Verification items for the finished model (mm, model axes). A direction names the side the tool comes from. Coordinates: 2 decimals unless noted, no trailing zeros. Write each loop counter-clockwise with the first axis right and the second up, starting at its lowest first coordinate (ties: lowest second). Pieces come first, ordered by that corner, then holes.
Autodesk Inventor part; units mm, degrees
ref_plane "Work Plane4" through (0, 32, 0) normal (0, 1, 0) x (-1, 0, 0)
ref_plane "YZ Plane" through (0, 0, 0) normal (1, 0, 0) x (0, 1, 0)
ref_plane "XY Plane" through (0, 0, 0) normal (0, 0, 1) x (1, 0, 0)
ref_plane "Work Plane4" through (0, 32, 0) normal (0, 1, 0) x (-1, 0, 0)
sketch "Sketch1" plane through (0, 0, 0) normal (0, 1, 0) x (-1, 0, 0)
  line L0 (33.75, 44.75) -> (-33.75, 44.75)
  line L1 (-33.75, 44.75) -> (-33.75, -44.75)
  line L2 (-33.75, -44.75) -> (33.75, -44.75)
  line L3 (33.75, -44.75) -> (33.75, 44.75)
  line L4 (21.75, -36.75) -> (-21.75, -36.75)
  line L5 (21.75, 36.75) -> (-21.75, 36.75)
  line L6 (21.75, 36.75) -> (21.75, -36.75)
  line L7 (-21.75, 36.75) -> (-21.75, -36.75)
  line L8 (33.75, -41.75) -> (-33.75, -41.75)
  line L9 (33.75, 41.75) -> (-33.75, 41.75)
  line L10 (-6.7955, 36.75) -> (21.75, 0)
  line L11 (21.75, 0) -> (0, -36.75)
  point P0 (0, 0)
  point P1 (-33.75, 0)
  dimension "d0" = 83.5
  dimension "d1" = 3
  dimension "d2" = 3
  dimension "d4" = 5
  dimension "d5" = 5
  dimension "d6" = 12
  dimension "d7" = 12
  dimension "d8" = 67.5
  dimension "d9" = 33.75
  dimension "d10" = 41.75
sketch "Sketch2" plane through (0, 32, 0) normal (0, 1, 0) x (1, 0, 0)
  line L0 (-65.75, 34.75) -> (24.75, 34.75)
  line L1 (-65.75, -34.75) -> (24.75, -34.75)
  line L2 (24.75, -34.75) -> (24.75, 34.75)
  line L3 (-65.75, -34.75) -> (-65.75, 34.75)
  line L4 (-74.75, -44.75) -> (-74.75, 44.75)
  line L5 (33.75, -44.75) -> (33.75, 44.75)
  line L6 (33.75, 44.75) -> (-33.75, 44.75)
  line L7 (-74.75, -44.75) -> (33.75, -44.75)
  line L8 (-74.75, 44.75) -> (33.75, 44.75)
  dimension "d94" = 69.5
  dimension "d96" = 90.5
  dimension "d97" = 9
  dimension "d98" = 9
  dimension "d99" = 10
  dimension "d100" = 10
extrude "Extrusion3" add sketch "Sketch2" along normal blind 3
sketch "Sketch3" plane through (0, 32, 0) normal (0, 1, 0) x (1, 0, 0)
  circle A0 centre (29.25, 0) radius 4.5
  circle A1 centre (-70.45, 0) radius 4.5
  circle A2 centre (-70.45, 0) radius 2.35
  circle A3 centre (29.25, 0) radius 2.35
  line L0 (33.75, -44.75) -> (33.75, 44.75)
  point P0 (0, 0)
  dimension "d24" = 9
  dimension "d27" = 4.7
  dimension "d43" = 99.7
  dimension "d44" = 4.5
extrude "Extrusion5" cut sketch "Sketch3" along normal blind 3 contours A2 | A3
sketch "Sketch9" plane through (0, 35, 0) normal (0, 1, 0) x (1, 0, 0)
  circle A0 centre (-39, -50.75) radius 3
  circle A1 centre (-39, -50.75) radius 6
  line L0 (-74.75, -44.75) -> (33.75, -44.75)
  circle A2 centre (-2, -50.75) radius 3
  circle A3 centre (-2, -50.75) radius 6
  arc A4 (7.1652, -44.75) -> (3.7885, -49.1711) centre (7.1652, -48.25) ccw
  arc A5 (-7.7885, -49.1711) -> (-11.1652, -44.75) centre (-11.1652, -48.25) ccw
  arc A6 (-29.8348, -44.75) -> (-33.2115, -49.1711) centre (-29.8348, -48.25) ccw
  arc A7 (-44.7885, -49.1711) -> (-48.1652, -44.75) centre (-48.1652, -48.25) ccw
  line L1 (33.75, -44.75) -> (33.75, 44.75)
  line L2 (-74.75, 44.75) -> (-74.75, -44.75)
  line L3 (64.0405, 0) -> (-151.031, 0) construction
  circle A8 centre (-39, 50.75) radius 3
  circle A9 centre (-39, 50.75) radius 6
  circle A10 centre (-2, 50.75) radius 3
  circle A11 centre (-2, 50.75) radius 6
  arc A12 (3.7885, 49.1711) -> (7.1652, 44.75) centre (7.1652, 48.25) ccw
  arc A13 (-11.1652, 44.75) -> (-7.7885, 49.1711) centre (-11.1652, 48.25) ccw
  arc A14 (-33.2115, 49.1711) -> (-29.8348, 44.75) centre (-29.8348, 48.25) ccw
  arc A15 (-48.1652, 44.75) -> (-44.7885, 49.1711) centre (-48.1652, 48.25) ccw
  line L4 (33.75, 44.75) -> (-74.75, 44.75)
  point P0 (0, 0)
  dimension "d101" = 6
  dimension "d102" = 12
  dimension "d103" = 37
  dimension "d104" = 7
  dimension "d105" = 108.5
  dimension "d106" = 35.75
extrude "Extrusion10" add sketch "Sketch9" against normal blind 3 contours A1 | A1 L0 A6 | A7 L0 A1 | L4 A11 A12 | A13 A11 L4 | A11
equation "\"d44\" = 0.5 * d24"
equation "\"d2\" = d1"
equation "\"d5\" = d4"
equation "\"d7\" = d6"
properties part number "CO-1-06-fuseMountTop"
1. Sectioned sample at B-B, the plane x = 29.25. Record the boundary of the cut face in (y, z), and give its area (3 significant figures).
2. Material ranges on L1, parallel to X at y = 34.45, z = 14; L2, parallel to Z at x = -2, y = 33.5; L3, parallel to X at y = 34, z = 0, recorded low to high.
3. Sectioned sample at C-C, the plane x = -39. Record the boundary of the cut face in (y, z).
4. Sectioned sample at A-A, the plane z = -50.75. Record the boundary of the cut face in (x, y), and give its area (3 significant figures).
5. Gauge pin test, flat end, axial feed: P1, Ø0.9, axis at x = 1.5, y = 33.5, coming from the -Z side. Record the tip position at first contact, or that the pin passes through.
6. Sectioned sample at D-D, the plane y = 34.55. Record the boundary of the cut face in (x, z).
7. Tool access check on faces 5 (the flat face through (24.75, 33, 0)), 6 (the flat face through (-43, 33, -44.75)), 7 (the flat face through (2, 33, 44.75)). Record the directions out of +Z, -Z, +X, -X, +Y, -Y that give a thin tool (end or side, any length) a straight path to the whole face; none if there is none.
8. Draft check along Z on faces 1 (the cylindrical face through (-8.41, 33.52, -46.09)), 2 (the cylindrical face through (-1.85, 33.52, -56.75)), 3 (the flat face through (20, 33, -44.75)), 4 (the flat face through (-74.75, 33, 1)). Enter one of: pulls with the +Z half, pulls with the -Z half, needs draft (parallel to the pull), parting line crosses it, or undercut.
Outcome:
1. outline: (32, -44.75) - (35, -44.75) - (35, -2.35) - (32, -2.35) - close; (32, 2.35) - (35, 2.35) - (35, 44.75) - (32, 44.75) - close
1. area: 254 mm2
2. L1: x = -74.75 to -65.75, 24.75 to 33.75
2. L2: z = -56.75 to -53.75, -47.75 to -34.75, 34.75 to 44.75
2. L3: x = -74.75 to -72.8, -68.1 to -65.75, 24.75 to 26.9, 31.6 to 33.75
3. outline: (32, -44.75) - (35, -44.75) - (35, -34.75) - (32, -34.75) - close; (32, 34.75) - (35, 34.75) - (35, 47.75) - (32, 47.75) - close; (32, 53.75) - (35, 53.75) - (35, 56.75) - (32, 56.75) - close
4. outline: (-8, 32) - (-5, 32) - (-5, 35) - (-8, 35) - close; (1, 32) - (4, 32) - (4, 35) - (1, 35) - close
4. area: 18.0 mm2
5. P1: stops at z = -55.92
6. outline: (-74.75, -44.75) - (-11.17, -44.75) arc R3.5 cw to (-7.79, -49.17) arc R6 ccw (long way) to (3.79, -49.17) arc R3.5 cw to (7.17, -44.75) - (33.75, -44.75) - (33.75, 44.75) - (-29.83, 44.75) arc R3.5 cw to (-33.21, 49.17) arc R6 ccw (long way) to (-44.79, 49.17) arc R3.5 cw to (-48.17, 44.75) - (-74.75, 44.75) - close; hole circle Ø4.7 at (-70.45, 0); hole (-65.75, -34.75) - (24.75, -34.75) - (24.75, 34.75) - (-65.75, 34.75) - close; hole circle Ø6 at (-39, 50.75); hole circle Ø6 at (-2, -50.75); hole circle Ø4.7 at (29.25, 0)
7. face 5: +Y, -Y
7. face 6: -Z, -X, +Y, -Y
7. face 7: +Z, +X, +Y, -Y
8. face 1: undercut
8. face 2: undercut
8. face 3: pulls with the -Z half
8. face 4: needs draft
